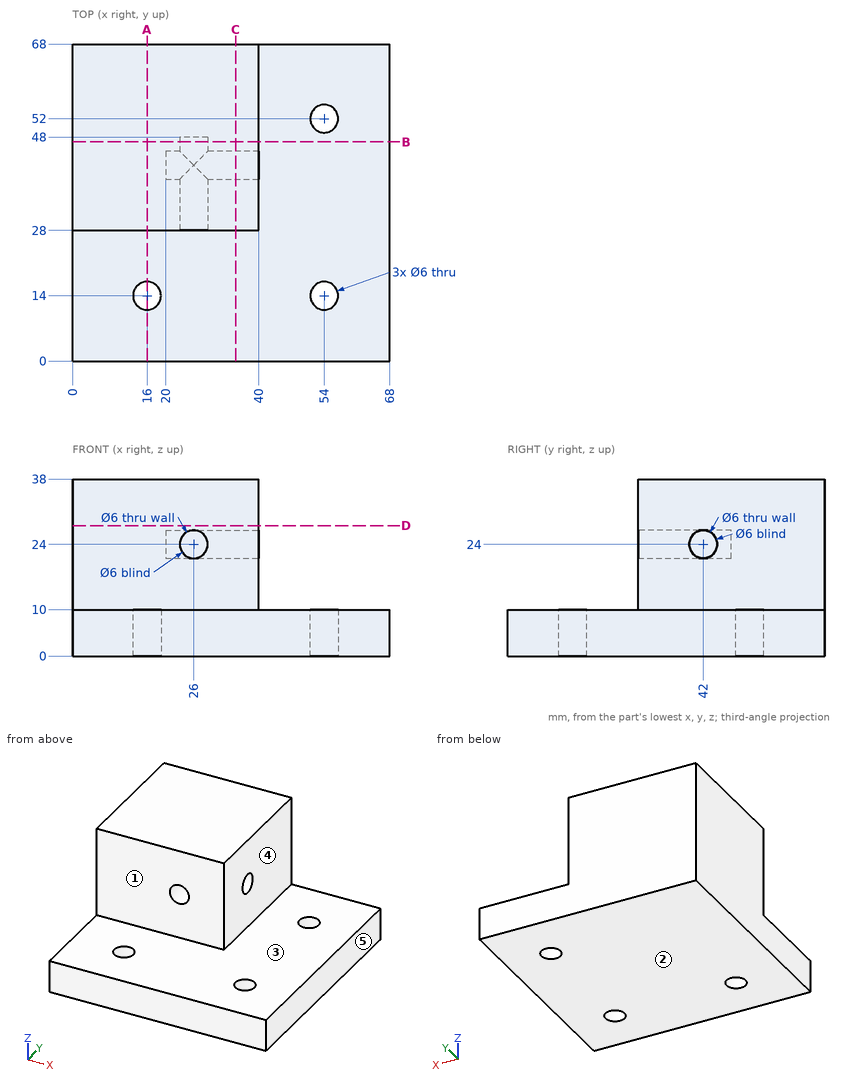
Geometry check sheet. Reference: drawing and pictorial views, mm from the part's lowest x, y, z. A direction names the side the tool comes from. Give positions to 0.01 mm unless a question says otherwise; leave off trailing zeros. Order: outer loops, then holes, each group sorted by start corner. A loop starts at its lowest first (then second) coordinate and runs counter-clockwise, first axis right, second up. Notation, with made-up numbers: M -36,87.25 L -1,87.25 A15 ccw -1,108.25 Z; hole C 45,-19 d1. An arc over 180 degrees is marked long. Return JSON: item names as keys, results as strings. Group by question number.
1) Section check C-C on x = 35. Record the cut outline in (y, z), and give its area (3 significant figures).
2) Section check D-D on z = 28. Record the cut outline in (x, y), and give its area (3 significant figures).
3) Section check B-B on y = 47. Record the cut outline in (x, z), and give its area (3 significant figures).
4) Scan lines: line 1 (Y direction, x = 53, z = 9); line 2 (Y direction, x = 21.45, z = 24); line 3 (X direction, y = 36.5, z = 16). Record each from-to range of solid material in increasing order.
5) Section check A-A on x = 16. Record the cut outline in (y, z), and give its area (3 significant figures).
6) Go/stop test with flat-tipped pins: pin 1 Ø6 at (x, z) = (32.5, 15.5) entering from -Y; pin 2 Ø22.5 at (y, z) = (55.5, 24.5) entering from +X; pin 3 Ø5.5 at (y, z) = (42, 24) entering from +X. Record where each tip stops, or that it passes through.
7) Access from +Z, -Z, +X, -X, +Y, -Y to the whole of each face (thin tool, end or side, straight path). Record for the marked faces 1, 2, 3, 4 and 5.
Answer block:
{
 "1": {"outline": "M 0,0 L 68,0 L 68,38 L 28,38 L 28,10 L 0,10 Z; hole C 42,24 d6", "area": "1,770 mm^2"},
 "2": {"outline": "M 0,28 L 40,28 L 40,68 L 0,68 Z", "area": "1,600 mm^2"},
 "3": {"outline": "M 0,0 L 68,0 L 68,10 L 40,10 L 40,38 L 0,38 Z; hole C 26,24 d6", "area": "1,770 mm^2"},
 "4": {"line 1": "y = 0 to 11.17, 16.83 to 49.17, 54.83 to 68", "line 2": "y = 28 to 39, 45 to 68", "line 3": "x = 0 to 40"},
 "5": {"outline": "M 0,0 L 11,0 L 11,10 L 0,10 Z; M 17,0 L 68,0 L 68,38 L 28,38 L 28,10 L 17,10 Z", "area": "1,740 mm^2"},
 "6": {"pin 1": "stops at y = 28", "pin 2": "stops at x = 40", "pin 3": "stops at x = 20"},
 "7": {"face 1": "+Z, +X, -X, -Y", "face 2": "-Z, +X, -X, +Y, -Y", "face 3": "+Z, +X, -Y", "face 4": "+Z, +X, +Y, -Y", "face 5": "+Z, -Z, +X, +Y, -Y"}
}
